```python
from build123d import *

# Parameters (mm, degrees)
BOSS_EXTRUDE1_DEPTH = 4


with BuildPart() as part:
    # Sketch1 → Boss-Extrude1 (new body)
    with BuildSketch(Plane.YZ):
        with BuildLine():
            Line((0, 0), (4, 0))
            Line((4, 0), (4, 3.556))
            Line((4, 3.556), (12.16, 3.556))
            ThreePointArc((12.16, 3.556), (15.752102448, 2.068102448), (17.24, -1.524))
            Line((17.24, -1.524), (17.24, -17.97))
            ThreePointArc((17.24, -17.97), (15.752102448, -21.562102448), (12.16, -23.05))
            Line((12.16, -23.05), (-0.54, -23.05))
            ThreePointArc((-0.54, -23.05), (-4.132102448, -21.562102448), (-5.62, -17.97))
            Line((-5.62, -17.97), (-5.62, -16.7))
            Line((-5.62, -16.7), (9.62, -16.7))
            Line((9.62, -16.7), (9.62, -12.7))
            Line((9.62, -12.7), (4, -12.7))
            Line((4, -12.7), (4, -7.62))
            Line((4, -7.62), (0, -7.62))
            Line((0, -7.62), (0, 0))
        make_face()
    extrude(amount=BOSS_EXTRUDE1_DEPTH)


solid = part.part
```
CAD build for the part. Positions are in the model's coordinates, mm. A direction names the side the tool comes from. Round coordinates to 2 decimals unless told otherwise and drop trailing zeros. Loops run counter-clockwise (first coordinate to the right, second up) from the corner with the lowest first, then second, coordinate; pieces in that order, holes last. Notation, with made-up numbers: M 54,-9 L 58,-9 A21 ccw 58,26 Z; hole C 46.25,63.5 d6. An arc over 180 degrees is marked long. Use a Markdown table: item, result. Add a question column.
(1) Cut at D-D (y = 3.5). Give the cut face in (x, z), and give its area (3 significant figures).
(2) Cut at B-B (x = 1.1). Give the cut face in (y, z), and give its area (3 significant figures).
(3) Cut at C-C (z = -8.5). Give the cut face in (x, y).
(4) Pull direction Z, two halves, no side cores. Call faces 4 (the face through (2, 8, 3.556)), 5 (the face through (2, 0, -4)), 6 (the face through (2, 9.62, -15)): +Z half, -Z half, draft (parallel to the pull), parting line (faces both ways), or undercut.
(5) Flat gauge pins, fed straight in: pin 1 (1.1 mm diameter, centred on x = 1.5, z = 2, fed in from -Y); pin 2 (1.5 mm diameter, centred on y = 4.5, z = -9.5, fed in from -X); pin 3 (2 mm diameter, centred on x = 1.5, y = 2, fed in from +Z). Where does each tip first touch, or does it go through?
(6) Drill centre lines: line 1 (Z direction, x = 1.6, y = 4.5); line 2 (Z direction, x = 1.3, y = 3.5); line 3 (Y direction, x = 3.45, z = -12.25). Where is each one in solid material? Low to high.
(7) Cut at A-A (y = 7.25). Give the cut face in (x, z), and give its area (3 significant figures).
(8) Which spindle directions (+Z, -Z, +X, -X, +Y, -Y) get a long thin tool onto all of the face, cutting with end or side? Do faces 1 (the face through (2, 7, -12.7)), 2 (the face through (2, -5.62, -17)), 3 (the face through (2, 2, 0)). Say none if no direction does.
Geometry says:
| question | item | result |
|---|---|---|
| 1 | outline | M 0,-23.05 L 4,-23.05 L 4,-16.7 L 0,-16.7 Z; M 0,-7.62 L 4,-7.62 L 4,0 L 0,0 Z |
| 1 | area | 55.9 mm² |
| 2 | outline | M -5.62,-17.97 A5.08 ccw -0.54,-23.05 L 12.16,-23.05 A5.08 ccw 17.24,-17.97 L 17.24,-1.52 A5.08 ccw 12.16,3.56 L 4,3.56 L 4,0 L 0,0 L 0,-7.62 L 4,-7.62 L 4,-12.7 L 9.62,-12.7 L 9.62,-16.7 L -5.62,-16.7 Z |
| 2 | area | 405 mm² |
| 3 | outline | M 0,4 L 4,4 L 4,17.24 L 0,17.24 Z |
| 4 | face 4 | +Z half |
| 4 | face 5 | draft |
| 4 | face 6 | undercut |
| 5 | pin 1 | stops at y = 4 |
| 5 | pin 2 | stops at x = 0 |
| 5 | pin 3 | stops at z = 0 |
| 6 | line 1 | z = -23.05 to -16.7, -12.7 to 3.56 |
| 6 | line 2 | z = -23.05 to -16.7, -7.62 to 0 |
| 6 | line 3 | y = 4 to 17.24 |
| 7 | outline | M 0,-23.05 L 4,-23.05 L 4,-16.7 L 0,-16.7 Z; M 0,-12.7 L 4,-12.7 L 4,3.56 L 0,3.56 Z |
| 7 | area | 90.4 mm² |
| 8 | face 1 | +X, -X, -Y |
| 8 | face 2 | +Z, -Z, +X, -X, -Y |
| 8 | face 3 | +Z, +X, -X, -Y |
